Source: three-view drawing plus pictorial views. Frame: mm from the lowest corner of the part. Give positions to 0.01 mm unless a question says otherwise; leave off trailing zeros. Loops run counter-clockwise (first coordinate to the right, second up) from the corner with the lowest first, then second, coordinate; pieces in that order, holes last.
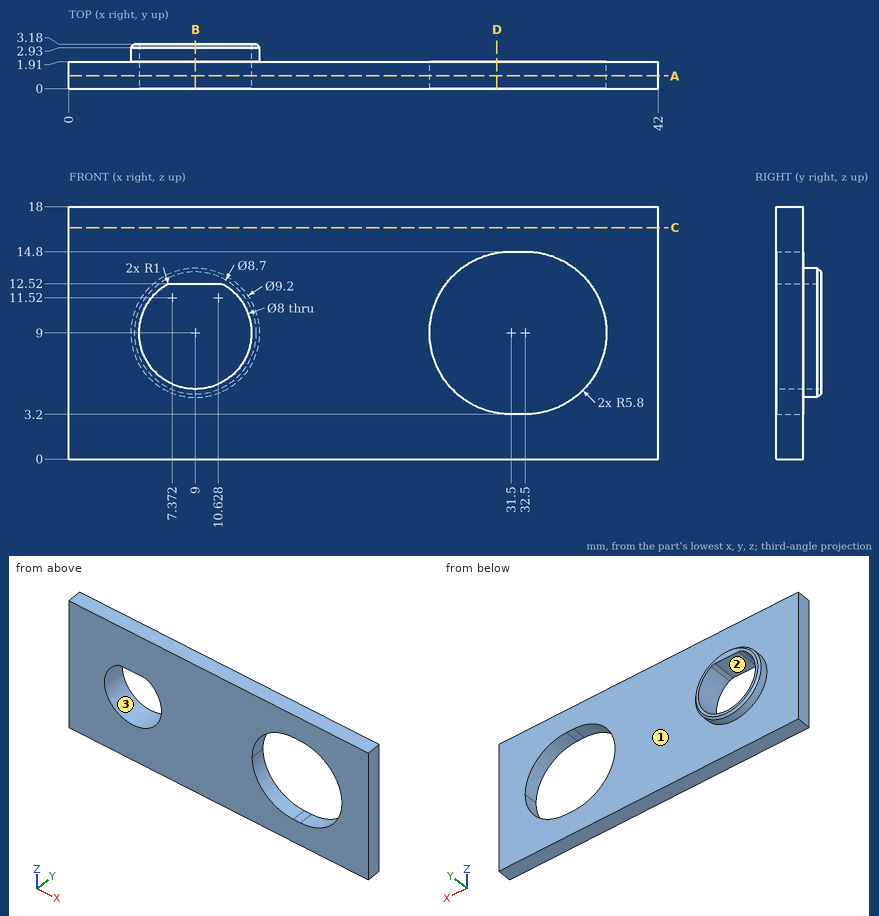
1) Cut plane C-C (z = 16.5). Return loops of the section in (x, y).
Checks:
outline: (0, 0) - (42, 0) - (42, 1.91) - (0, 1.91) - close
2) Cut plane D-D (x = 30.5). Return loops of the section in (y, z).
Checks:
outline: (0, 0) - (1.91, 0) - (1.91, 3.29) - (0, 3.29) - close; (0, 14.71) - (1.91, 14.71) - (1.91, 18) - (0, 18) - close
3) Cut plane B-B (x = 9). Return loops of the section in (y, z), and give its area (3 significant figures).
Checks:
outline: (0, 0) - (1.91, 0) - (1.91, 4.4) - (2.93, 4.4) - (3.18, 4.65) - (3.18, 5) - (0, 5) - close; (0, 12.52) - (3.18, 12.52) - (3.18, 13.35) - (2.93, 13.6) - (1.91, 13.6) - (1.91, 18) - (0, 18) - close
area: 22.1 mm2
4) Contact query for a flat-ended pin moving along its axis: P1, Ø9, axis at x = 15.5, z = 5, coming from the +Y side. Output: stop coordinate, or through.
Checks:
P1: stops at y = 3.18
5) Ray query, probe 1 along X at (y, z) = (1, 9); probe 2 along X at (y, z) = (1.75, 11.75) (1 decimal); probe 3 along X at (y, z) = (2.1, 7.25) (1 decimal). Return the intervals inside material, ascending.
Checks:
probe 1: x = 0 to 5, 13 to 25.7, 38.3 to 42
probe 2: x = 0 to 6.1, 11.9 to 26.4, 37.6 to 42
probe 3: x = 4.7 to 5.4, 12.6 to 13.3
6) Cut plane A-A (y = 0.9). Return loops of the section in (x, z).
Checks:
outline: (0, 0) - (42, 0) - (42, 18) - (0, 18) - close; hole (6.83, 12.36) arc R4 ccw (long way) to (11.17, 12.36) arc R1 ccw to (10.63, 12.52) - (7.37, 12.52) arc R1 ccw to start; hole (31.5, 3.2) - (32.5, 3.2) arc R5.8 ccw to (32.5, 14.8) - (31.5, 14.8) arc R5.8 ccw to start
7) Pull-direction query (X, two-part tool) for the marked faces 1, 2 and 3; classes: released by +X, released by -X, zero draft, split by the parting line, or undercut.
Checks:
face 1: zero draft
face 2: undercut
face 3: undercut
